from build123d import *

# Parameters (mm, degrees)
SKETCH1_R                            = 4
BOSS_EXTRUDE1_DEPTH                  = 34
F_3_2_3_2_DIAMETER_HOLE3_D           = 3.2
F_3_2_3_2_DIAMETER_HOLE3_DEPTH       = 14
F_3_2_3_2_DIAMETER_HOLE3_CSINK_D     = 3.25
F_3_2_3_2_DIAMETER_HOLE3_CSINK_ANGLE = 90
F_3_2_3_2_DIAMETER_HOLE3_TIP         = 0.96137699
SKETCH4_W                            = 3
SKETCH4_H                            = 4
SKETCH4_H_2                          = 12
CUT_EXTRUDE1_DEPTH                   = 4
SKETCH8_R                            = 2
BOSS_EXTRUDE2_DEPTH                  = 12
SKETCH9_R                            = 2
BOSS_EXTRUDE3_DEPTH                  = 0.5
BOSS_EXTRUDE3_TAPER                  = 45


with BuildPart() as part:
    # Sketch1 → Boss-Extrude1 (new body)
    with BuildSketch(Plane(origin=(0, 0, 0), x_dir=(1, 0, 0), z_dir=(0, 1, 0))):
        with Locations(Location((0, 0, 0), (0, 0, 270))):
            Circle(SKETCH1_R)
    extrude(amount=BOSS_EXTRUDE1_DEPTH)

    # Ø3.2 (3.2) Diameter Hole3
    with Locations(Plane(origin=(0, 0, 0), x_dir=(-1, 0, 0), z_dir=(0, -1, 0))):
        with Locations((0, 0)):
            CounterSinkHole(F_3_2_3_2_DIAMETER_HOLE3_D / 2, F_3_2_3_2_DIAMETER_HOLE3_CSINK_D / 2, depth=F_3_2_3_2_DIAMETER_HOLE3_DEPTH, counter_sink_angle=F_3_2_3_2_DIAMETER_HOLE3_CSINK_ANGLE)
            with Locations((0, 0, -(F_3_2_3_2_DIAMETER_HOLE3_DEPTH + F_3_2_3_2_DIAMETER_HOLE3_TIP / 2))):  # 118° drill point
                Cone(0, F_3_2_3_2_DIAMETER_HOLE3_D / 2, F_3_2_3_2_DIAMETER_HOLE3_TIP, mode=Mode.SUBTRACT)

    # Sketch4 → Cut-Extrude1 (cut, symmetric)
    with BuildSketch(Plane(origin=(0, 0, 0), x_dir=(0, 0, -1), z_dir=(1, 0, 0))):
        with Locations((-4, 11.5)):
            Rectangle(SKETCH4_W, SKETCH4_H)
        with Locations((4, 15.5)):
            Rectangle(SKETCH4_W, SKETCH4_H_2)
    extrude(amount=CUT_EXTRUDE1_DEPTH, both=True, mode=Mode.SUBTRACT)

    # Sketch6 → Ø4.0 (4) Diameter Hole2 (revolve, cut)
    with BuildSketch(Plane(origin=(0, 11.5, 2.5), x_dir=(0, -1, 0), z_dir=(1, 0, 0))):
        Polygon((0, 0), (0, 2.5), (2, 1.298278762), (2, 0.025), (2.025, 0), align=None)
    revolve(axis=Axis((0, 11.5, 8.85), (0, 0, -1)), mode=Mode.SUBTRACT)

    # Sketch8 → Boss-Extrude2 (add)
    with BuildSketch(Plane(origin=(0, 34, 0), x_dir=(1, 0, 0), z_dir=(0, 1, 0))):
        with Locations(Location((0, 0, 0), (0, 0, 270))):
            Circle(SKETCH8_R)
    extrude(amount=BOSS_EXTRUDE2_DEPTH)

    # Sketch9 → Boss-Extrude3 (add)
    with BuildSketch(Plane(origin=(0, 46, 0), x_dir=(1, 0, 0), z_dir=(0, 1, 0))):
        with Locations(Location((0, 0, 0), (0, 0, 270))):
            Circle(SKETCH9_R)
    extrude(amount=BOSS_EXTRUDE3_DEPTH, taper=BOSS_EXTRUDE3_TAPER)


solid = part.part
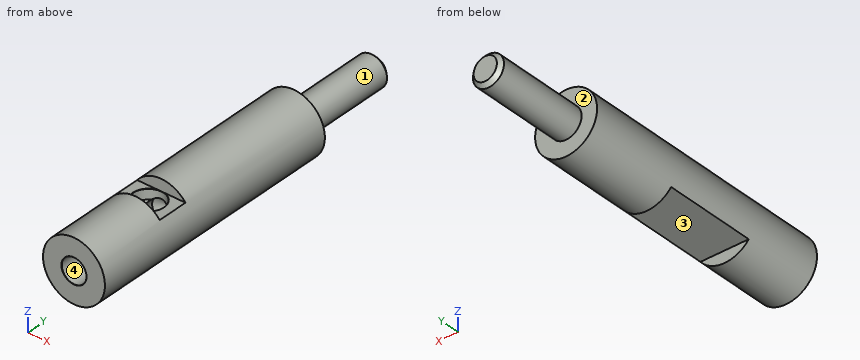
Design review of the part built by this model. Coordinates are the model's own, in mm. Face numbers are marked on the shaded views. Give positions to 0.01 mm unless a question says otherwise; leave off trailing zeros. Order: outer loops, then holes, each group sorted by start corner. A loop starts at its lowest first (then second) coordinate and runs counter-clockwise, first axis right, second up.
1. Add section B-B, the plane y = 33. State the section outline as (x, z) points, then the cut area to 3 significant figures.
Solution:
outline: circle Ø8 at (0, 0)
area: 50.3 mm2
2. To check wall thickness, follow L1, parallel to X at y = 25.5, z = 2.5; L2, parallel to Z at x = 2.5, y = 14; L3, parallel to Y at x = 3.25, z = 2.25. State the ranges of each line that lie inside material, in increasing order.
Solution:
L1: x = -3.12 to 3.12
L2: z = -2.5 to 3.12
L3: y = 0 to 34
3. Add section D-D, the plane y = 39. State the section outline as (x, z) points.
Solution:
outline: circle Ø4 at (0, 0)
4. Mouldability with a two-part tool opening along Z and no side actions: class the marked faces 1, 2, 3 and 4 as +Z half, -Z half, draft (parallel to the pull), parting line (faces both ways), or undercut.
Solution:
face 1: parting line
face 2: draft
face 3: -Z half
face 4: undercut
5. For pin 1 Ø1.9 at (x, y) = (1.5, 13) entering from -Z; pin 2 Ø0.8 at (x, z) = (0.5, -3.5) entering from +Y; pin 3 Ø3.5 at (x, y) = (0, 11.5) entering from +Z; pin 4 Ø0.8 at (x, z) = (1.5, 3) entering from -Y, all flat-tipped, find the tip position at first contact; note any pin that passes through.
Solution:
pin 1: stops at z = -2.5
pin 2: stops at y = 34
pin 3: stops at z = 1.05
pin 4: stops at y = 0
6. Add section A-A, the plane y = 18. State the section outline as (x, z) points.
Solution:
outline: (-3.12, -2.5) - (3.12, -2.5) arc R4 ccw (long way) to start
